Check sheet for the modelled part. Datum: model origin and axes. Units: mm. A direction names the side the tool comes from. Coordinates: 2 decimals unless noted, no trailing zeros. Loops run counter-clockwise (first coordinate to the right, second up) from the corner with the lowest first, then second, coordinate; pieces in that order, holes last. Notation, with made-up numbers: (8.25, 38.5) -> (59.25, 38.5) arc R13 cw to (59.25, 42.5) -> close; hole circle Ø4 at (-15, 53). An arc over 180 degrees is marked (long way). Use CSV: the item, a comma, the result in double quotes. Start each with the question number.
1. Release check for a two-part mould opening along Y. For faces 5 (the face through (-8, 1, 19.85)), 6 (the face through (23.674, 9.712, 11.92)), 7 (the face through (-18, 14, 16.85)) record: pulls with the +Y half, pulls with the -Y half, needs draft (parallel to the pull), parting line crosses it, or undercut.
2. Sectioned sample at B-B, the plane x = -20. Record the cut outline in (y, z).
3. Sectioned sample at A-A, the plane z = 12.75. Count the separate pieces of the cut face and the enclosed holes in it, and give its area (3 significant figures).
4. Thickness scan on L1, parallel to Y at x = 0, z = 0.7 (3 decimals); L2, parallel to Y at x = 0, z = 19.1 (3 decimals); L3, parallel to X at y = 22, z = 13.25. Record the ranges inside material, lowest first.
5. Set-up check for faces 1 (the face through (-26, 1, 6.85)), 2 (the face through (-1.005, -7.654, 1.521)), 3 (the face through (-1.525, 0, 10)), 4 (the face through (2, 0, 19.85)): record each of +Z, -Z, +X, -X, +Y, -Y from which the full face is reachable in a straight line by a thin tool's end or side.
6. Gauge pin test, flat ends, axial feed: pin 1 (1 mm diameter, centred on x = -37.5, z = 12, fed in from +Y); pin 2 (8 mm diameter, centred on y = 40.5, z = 16.5, fed in from +X); pin 3 (8.5 mm diameter, centred on x = -13.5, y = 11.5, fed in from +Z). Record the tip position at first contact, or that the pin passes through.
```python
from build123d import *
from build123d.topology import SkipClean

# Parameters (mm, degrees)
SKETCH1_R           = 50.8
SKETCH1_R_2         = 8.57
SKETCH1_R_3         = 7.72
SKETCH1_R_4         = 5.275
SKETCH1_W           = 3.05
SKETCH1_H           = 3.05
BOSS_EXTRUDE1_DEPTH = 19.85
SKETCH2_R           = 7.72
SKETCH2_R_2         = 5.275
CUT_EXTRUDE1_DEPTH  = 3
SKETCH3_R           = 40.74
SKETCH3_R_2         = 8.57
CUT_EXTRUDE2_DEPTH  = 3
CUT_EXTRUDE3_START  = -3
SKETCH4_R           = 45.337827748
SKETCH4_R_2         = 8.57
SKETCH4_R_3         = 7.72
SKETCH4_R_4         = 5.275
CUT_EXTRUDE3_DEPTH  = 3
CUT_EXTRUDE4_DEPTH  = 10


with BuildPart() as part:
    # Sketch1 → Boss-Extrude1 (new body)
    # profile 1 of 4: a face of its own
    with BuildSketch(Plane.XY):
        Circle(SKETCH1_R)
        Circle(SKETCH1_R_2, mode=Mode.SUBTRACT)
    # profile 2 of 4: a face of its own
    with BuildSketch(Plane.XY):
        Circle(SKETCH1_R_2)
        Circle(SKETCH1_R_3, mode=Mode.SUBTRACT)
    # profile 3 of 4: a face of its own
    with BuildSketch(Plane.XY):
        Circle(SKETCH1_R_3)
        Circle(SKETCH1_R_4, mode=Mode.SUBTRACT)
    # profile 4 of 4: a face of its own
    with BuildSketch(Plane.XY):
        Circle(SKETCH1_R_4)
        Rectangle(SKETCH1_W, SKETCH1_H, mode=Mode.SUBTRACT)
    extrude(amount=BOSS_EXTRUDE1_DEPTH)

    # Sketch2 → Cut-Extrude1 (cut)
    with BuildSketch(Plane.XY.offset(19.85)):
        Circle(SKETCH2_R)
        Circle(SKETCH2_R_2, mode=Mode.SUBTRACT)
    extrude(amount=-CUT_EXTRUDE1_DEPTH, mode=Mode.SUBTRACT)

    # Sketch3 → Cut-Extrude2 (cut)
    with BuildSketch(Plane.XY.offset(19.85)):
        Circle(SKETCH3_R)
        Circle(SKETCH3_R_2, mode=Mode.SUBTRACT)
    extrude(amount=-CUT_EXTRUDE2_DEPTH, mode=Mode.SUBTRACT)

    # Sketch4 → Cut-Extrude3 (cut)
    # profile 1 of 2: a face of its own
    with BuildSketch(Plane(origin=(0, 0, 0), x_dir=(-1, 0, 0), z_dir=(0, 0, -1)).offset(CUT_EXTRUDE3_START)):
        Circle(SKETCH4_R)
        with Locations(Location((0, 0, 0), (0, 0, 180))):
            Circle(SKETCH4_R_2, mode=Mode.SUBTRACT)
    # profile 2 of 2: a face of its own
    with BuildSketch(Plane(origin=(0, 0, 0), x_dir=(-1, 0, 0), z_dir=(0, 0, -1)).offset(CUT_EXTRUDE3_START)):
        with Locations(Location((0, 0, 0), (0, 0, 180))):
            Circle(SKETCH4_R_3)
        with Locations(Location((0, 0, 0), (0, 0, 180))):
            Circle(SKETCH4_R_4, mode=Mode.SUBTRACT)
    extrude(amount=CUT_EXTRUDE3_DEPTH, mode=Mode.SUBTRACT)

    # Sketch5 → Cut-Extrude4 (cut)
    with SkipClean():  # the faces are left unmerged after this step: merging them gives an invalid solid
        with BuildSketch(Plane.XY.offset(16.85)):
            with BuildLine():
                ThreePointArc((-40.155721572, 6.875), (-19.932515852, 15.660919221), (0.928253594, 8.519580111))
                ThreePointArc((0.928253594, 8.519580111), (3.182932587, 7.956999444), (5.20358481, 6.809376265))
                ThreePointArc((5.20358481, 6.809376265), (0.190794067, 25.869806658), (-15.630243014, 37.622375036))
                ThreePointArc((-15.630243014, 37.622375036), (-31.849155862, 25.404308117), (-40.155721572, 6.875))
            make_face()
            with BuildLine():
                ThreePointArc((-14.123936135, 38.213374989), (3.596495966, 25.0925247), (7.842299603, 3.455898861))
                ThreePointArc((7.842299603, 3.455898861), (8.386101824, 1.7658415), (8.57, 0))
                ThreePointArc((8.57, 0), (8.552202829, -0.552020624), (8.498885235, -1.101748504))
                ThreePointArc((8.498885235, -1.101748504), (22.499306791, 12.76967082), (24.766811024, 32.347375036))
                ThreePointArc((24.766811024, 32.347375036), (6.076198264, 40.284332124), (-14.123936135, 38.213374989))
            make_face()
            with BuildLine():
                ThreePointArc((6.914046008, -5.063681249), (5.299497363, -6.735000201), (3.295300425, -7.911124769))
                ThreePointArc((3.295300425, -7.911124769), (22.308512723, -13.100135838), (40.397054039, -5.275))
                ThreePointArc((40.397054039, -5.275), (40.654173104, -2.643068148), (40.74, 0))
                ThreePointArc((40.74, 0), (36.880093131, 17.30914009), (26.031785437, 31.338374989))
                ThreePointArc((26.031785437, 31.338374989), (23.529011818, 9.431605478), (6.914046008, -5.063681249))
            make_face()
            with BuildLine():
                ThreePointArc((-0.928253594, -8.519580111), (-3.182932587, -7.956999444), (-5.20358481, -6.809376265))
                ThreePointArc((-5.20358481, -6.809376265), (-0.190794067, -25.869806658), (15.630243014, -37.622375036))
                ThreePointArc((15.630243014, -37.622375036), (31.849155862, -25.404308117), (40.155721572, -6.875))
                ThreePointArc((40.155721572, -6.875), (19.932515852, -15.660919221), (-0.928253594, -8.519580111))
            make_face()
            with BuildLine():
                ThreePointArc((-7.842299603, -3.455898861), (-8.48242995, -1.221999243), (-8.498885235, 1.101748504))
                ThreePointArc((-8.498885235, 1.101748504), (-22.499306791, -12.76967082), (-24.766811024, -32.347375036))
                ThreePointArc((-24.766811024, -32.347375036), (-6.076198264, -40.284332124), (14.123936135, -38.213374989))
                ThreePointArc((14.123936135, -38.213374989), (-3.596495966, -25.0925247), (-7.842299603, -3.455898861))
            make_face()
            with BuildLine():
                ThreePointArc((-6.914046008, 5.063681249), (-5.299497363, 6.735000201), (-3.295300425, 7.911124769))
                ThreePointArc((-3.295300425, 7.911124769), (-22.308512723, 13.100135838), (-40.397054039, 5.275))
                ThreePointArc((-40.397054039, 5.275), (-37.925354126, -14.880024007), (-26.031785437, -31.338374989))
                ThreePointArc((-26.031785437, -31.338374989), (-23.529011818, -9.431605478), (-6.914046008, 5.063681249))
            make_face()
        extrude(amount=-CUT_EXTRUDE4_DEPTH, mode=Mode.SUBTRACT)


solid = part.part
```
Completed:
1,face 5,"needs draft"
1,face 6,"undercut"
1,face 7,"undercut"
2,outline,"(-46.7, 0) -> (-40.69, 0) -> (-40.69, 3) -> (40.69, 3) -> (40.69, 0) -> (46.7, 0) -> (46.7, 19.85) -> (35.49, 19.85) -> (35.49, 6.85) -> (15.66, 6.85) -> (15.66, 16.85) -> (13.17, 16.85) -> (13.17, 6.85) -> (-4.14, 6.85) -> (-4.14, 16.85) -> (-8.55, 16.85) -> (-8.55, 6.85) -> (-35.49, 6.85) -> (-35.49, 19.85) -> (-46.7, 19.85) -> close"
3,separate pieces,"1"
3,enclosed holes,"7"
3,area,"3,700 mm²"
4,L1,"-50.8 to -45.338, -8.57 to -7.72, -5.275 to -1.525, 1.525 to 5.275, 7.72 to 8.57, 45.338 to 50.8"
4,L2,"-50.8 to -40.74, -8.57 to -7.72, -5.275 to -1.525, 1.525 to 5.275, 7.72 to 8.57, 40.74 to 50.8"
4,L3,"-45.79 to -34.29, 2.4 to 5.31, 25.26 to 26.98, 34.29 to 45.79"
5,face 1,"+Z"
5,face 2,"-Z"
5,face 3,"+Z, -Z"
5,face 4,"+Z, +X, -X, +Y, -Y"
6,pin 1,"y = 34.81"
6,pin 2,"x = 35.33"
6,pin 3,"z = 16.85"
